The listing builds one solid part. Answer for the finished solid, in the listing's coordinates (mm). Give positions to 0.01 mm unless a question says otherwise; leave off trailing zeros. Order: outer loops, then holes, each group sorted by start corner. A loop starts at its lowest first (then second) coordinate and runs counter-clockwise, first axis right, second up. Notation, with made-up numbers: (35.5, -34) -> (92.5, -34) arc R5 cw to (92.5, -28) -> close; hole circle Ø6 at (57.25, -36.75). An arc over 180 degrees is marked (long way). Answer as a JSON object with one key per item and string values. Group by question number.
```python
from build123d import *

# Parameters (mm, degrees)
SKETCH1_R           = 1.625
SKETCH1_R_2         = 2.5
SKETCH1_R_3         = 1.65
SKETCH1_W           = 8
SKETCH1_H           = 30
SKETCH1_W_2         = 5
SKETCH1_H_2         = 15
BOSS_EXTRUDE1_DEPTH = 8
FILLET1_R           = 10
CUT_EXTRUDE1_DEPTH  = 9


with BuildPart() as part:
    # Sketch1 → Boss-Extrude1 (new body)
    with BuildSketch(Plane.XY):
        Polygon((70, 380), (250, 380), (250, 415), (320, 415), (320, 0), (0, 0), (0, 415), (70, 415), align=None)
        with Locations((14, 388)):
            Circle(SKETCH1_R, mode=Mode.SUBTRACT)
        with Locations((36, 388)):
            Circle(SKETCH1_R, mode=Mode.SUBTRACT)
        with Locations((41, 362.5)):
            Circle(SKETCH1_R_2, mode=Mode.SUBTRACT)
        with Locations((279, 362.5)):
            Circle(SKETCH1_R_2, mode=Mode.SUBTRACT)
        with Locations((284, 388)):
            Circle(SKETCH1_R, mode=Mode.SUBTRACT)
        with Locations((306, 388)):
            Circle(SKETCH1_R, mode=Mode.SUBTRACT)
        with Locations((239, 365)):
            Circle(SKETCH1_R_3, mode=Mode.SUBTRACT)
        with Locations((81, 365)):
            Circle(SKETCH1_R_3, mode=Mode.SUBTRACT)
        with Locations((239, 305)):
            Circle(SKETCH1_R_3, mode=Mode.SUBTRACT)
        with Locations((81, 305)):
            Circle(SKETCH1_R_3, mode=Mode.SUBTRACT)
        with Locations((239, 245)):
            Circle(SKETCH1_R_3, mode=Mode.SUBTRACT)
        with Locations((81, 245)):
            Circle(SKETCH1_R_3, mode=Mode.SUBTRACT)
        with Locations((239, 185)):
            Circle(SKETCH1_R_3, mode=Mode.SUBTRACT)
        with Locations((81, 185)):
            Circle(SKETCH1_R_3, mode=Mode.SUBTRACT)
        with Locations((239, 125)):
            Circle(SKETCH1_R_3, mode=Mode.SUBTRACT)
        with Locations((81, 125)):
            Circle(SKETCH1_R_3, mode=Mode.SUBTRACT)
        with Locations((239, 65)):
            Circle(SKETCH1_R_3, mode=Mode.SUBTRACT)
        with Locations((81, 65)):
            Circle(SKETCH1_R_3, mode=Mode.SUBTRACT)
        with Locations((81, 35)):
            Rectangle(SKETCH1_W, SKETCH1_H, mode=Mode.SUBTRACT)
        with Locations((30.5, 362.5)):
            Rectangle(SKETCH1_W_2, SKETCH1_H_2, mode=Mode.SUBTRACT)
        with Locations((51.5, 362.5)):
            Rectangle(SKETCH1_W_2, SKETCH1_H_2, mode=Mode.SUBTRACT)
        with Locations((268.5, 362.5)):
            Rectangle(SKETCH1_W_2, SKETCH1_H_2, mode=Mode.SUBTRACT)
        with Locations((289.5, 362.5)):
            Rectangle(SKETCH1_W_2, SKETCH1_H_2, mode=Mode.SUBTRACT)
        with Locations((239, 35)):
            Rectangle(SKETCH1_W, SKETCH1_H, mode=Mode.SUBTRACT)
        with Locations((81, 95)):
            Rectangle(SKETCH1_W, SKETCH1_H, mode=Mode.SUBTRACT)
        with Locations((239, 95)):
            Rectangle(SKETCH1_W, SKETCH1_H, mode=Mode.SUBTRACT)
        with Locations((81, 155)):
            Rectangle(SKETCH1_W, SKETCH1_H, mode=Mode.SUBTRACT)
        with Locations((239, 155)):
            Rectangle(SKETCH1_W, SKETCH1_H, mode=Mode.SUBTRACT)
        with Locations((81, 215)):
            Rectangle(SKETCH1_W, SKETCH1_H, mode=Mode.SUBTRACT)
        with Locations((239, 215)):
            Rectangle(SKETCH1_W, SKETCH1_H, mode=Mode.SUBTRACT)
        with Locations((81, 275)):
            Rectangle(SKETCH1_W, SKETCH1_H, mode=Mode.SUBTRACT)
        with Locations((239, 275)):
            Rectangle(SKETCH1_W, SKETCH1_H, mode=Mode.SUBTRACT)
        with Locations((81, 335)):
            Rectangle(SKETCH1_W, SKETCH1_H, mode=Mode.SUBTRACT)
        with Locations((239, 335)):
            Rectangle(SKETCH1_W, SKETCH1_H, mode=Mode.SUBTRACT)
    extrude(amount=BOSS_EXTRUDE1_DEPTH)

    # Fillet1
    fillet1_edges = [part.edges().sort_by_distance(p)[0] for p in [
        (0, 415, 4),
        (70, 415, 4),
        (70, 380, 4),
        (250, 380, 4),
        (250, 415, 4),
        (320, 415, 4),
    ]]
    fillet(fillet1_edges, radius=FILLET1_R)

    # Sketch2 → Cut-Extrude1 (cut, through all)
    with BuildSketch(Plane.XY.offset(8)):
        with BuildLine():
            Line((127.5, 330), (192.5, 330))
            ThreePointArc((192.5, 330), (202.5, 320), (192.5, 310))
            Line((192.5, 310), (127.5, 310))
            ThreePointArc((127.5, 310), (117.5, 320), (127.5, 330))
        make_face()
    extrude(amount=-CUT_EXTRUDE1_DEPTH, mode=Mode.SUBTRACT)


solid = part.part
```
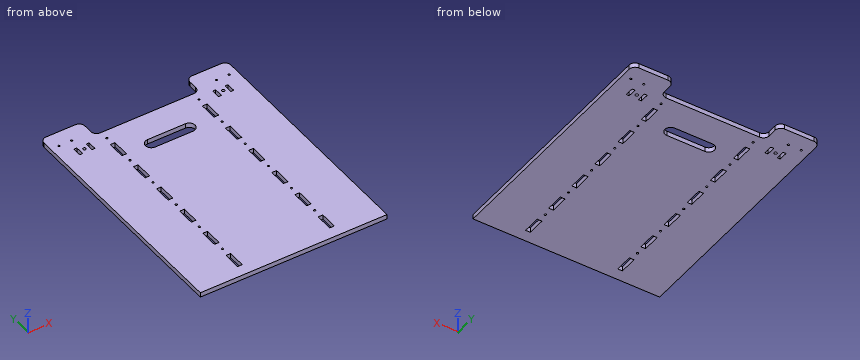
(1) Find the intervals of material crossed by line 1 along X through (y, z) = (245, 2.25); line 2 along X through (y, z) = (349, 2.75); line 3 along Y through (x, z) = (137.5, 3), in increasing order. Write a range as [from, to].
(2) A cutting plane is placed at B-B (x = 181.5). Determine the outline of the cut face in (y, z).
(3) Flat-ended cylindrical pins translate along their axes: pin 1 Ø4 at (x, z) = (153.5, 3) entering from +Y; pin 2 Ø2.5 at (x, z) = (79, 2.5) entering from +Y; pin 3 Ø3 at (x, z) = (116, 6.5) entering from -Y. Find the tip coordinate at first contact, or state that the pin passes through.
(4) A cutting plane is placed at A-A (y = 337). Determine the outline of the cut face in (x, z), and give its area (3 significant figures).
(5) A cutting plane is placed at C-C (z = 2.5). State how many separate pieces and enclosed holes the cut face has, and give its area (3 significant figures).
Check sheet entries:
{
 "1": {"line 1": "x = [0, 79.35], [82.65, 237.35], [240.65, 320]", "line 2": "x = [0, 77], [85, 235], [243, 320]", "line 3": "y = [0, 310], [330, 380]"},
 "2": {"outline": "(0, 0) -> (310, 0) -> (310, 8) -> (0, 8) -> close; (330, 0) -> (380, 0) -> (380, 8) -> (330, 8) -> close"},
 "3": {"pin 1": "stops at y = 380", "pin 2": "stops at y = 380.26", "pin 3": "stops at y = 0"},
 "4": {"outline": "(0, 0) -> (77, 0) -> (77, 8) -> (0, 8) -> close; (85, 0) -> (235, 0) -> (235, 8) -> (85, 8) -> close; (243, 0) -> (320, 0) -> (320, 8) -> (243, 8) -> close", "area": "2,430 mm2"},
 "5": {"separate pieces": "1", "enclosed holes": "35", "area": "121,000 mm2"}
}
